Part model, mm, in its own coordinate system. A direction names the side the tool comes from. Coordinates: 2 decimals unless noted, no trailing zeros. Loops run counter-clockwise (first coordinate to the right, second up) from the corner with the lowest first, then second, coordinate; pieces in that order, holes last. Notation, with made-up numbers: M 2,57.5 L 44,57.5 A18 ccw 44,63.5 Z; hole C 53.25,20 d2. An arc over 180 degrees is marked long. Use a Markdown table: item, result. Add a question column.
1) Band-saw the part on A-A (z = 0). List the corners of the cut face in (x, y).
2) Pull direction X, two halves, no side cores. Call faces 1 (the flat face through (-25, -45, 0)), 2 (the flat face through (-12, -70, 0)), 3 (the flat face through (-13, -45, 10)), 4 (the flat face through (0, -32, 0)): released by +X, released by -X, zero draft, split by the parting line, or undercut.
3) Band-saw the part on D-D (z = 5.25). List the corners of the cut face in (x, y), plus the area to 3 significant figures.
4) Band-saw the part on C-C (y = -22.5). List the corners of the cut face in (x, z).
5) Wall check: probe 1 along X at (y, z) = (-73, 0); probe 2 along Z at (x, y) = (-12, -74); probe 3 along Z at (x, y) = (-15.5, -28). Give the ranges that are in metal, low to high. Write a range as from..to.
6) Band-saw the part on B-B (x = -12.5). List the corners of the cut face in (y, z), plus the area to 3 significant figures.
7) Pin check, flat tips, straight feed: pin 1 Ø12 at (x, y) = (-14.5, -48) entering from +Z; pin 2 Ø10 at (y, z) = (-30.5, 0) entering from -X; pin 3 Ø5.5 at (x, z) = (-14, -1) entering from -Y. Stop position of each tip, or through.
8) Tool access for faces 5 (the flat face through (-13, -45, -10)), 6 (the cylindrical face through (-21.286, -75.07, 1.951)), 7 (the flat face through (-10, -80, -9)): list every direction of +Z, -Z, +X, -X, +Y, -Y with a clear straight run to the whole face (end or side of a thin tool).
from build123d import *

# Parameters (mm, degrees)
SKETCH1_R           = 15
BOSS_EXTRUDE1_DEPTH = 50
SKETCH2_W           = 25
SKETCH2_H           = 20
BOSS_EXTRUDE2_DEPTH = 80
SKETCH3_R           = 9
CUT_EXTRUDE2_DEPTH  = 10


with BuildPart() as part:
    # Sketch1 → Boss-Extrude1 (new body)
    with BuildSketch(Plane(origin=(0, 0, 0), x_dir=(0, 0, -1), z_dir=(1, 0, 0))):
        Circle(SKETCH1_R)
    extrude(amount=-BOSS_EXTRUDE1_DEPTH)

    # Sketch2 → Boss-Extrude2 (add)
    with BuildSketch(Plane(origin=(0, 0, 0), x_dir=(1, 0, 0), z_dir=(0, 1, 0))):
        with Locations((-12.5, 0)):
            Rectangle(SKETCH2_W, SKETCH2_H)
    extrude(amount=-BOSS_EXTRUDE2_DEPTH)

    # Sketch3 → Cut-Extrude2 (cut)
    with BuildSketch(Plane.XZ.offset(80)):
        with Locations(Location((-12.5, 0, 0), (0, 0, 270))):
            Circle(SKETCH3_R)
    extrude(amount=-CUT_EXTRUDE2_DEPTH, mode=Mode.SUBTRACT)


solid = part.part
Entries:
| question | item | result |
|---|---|---|
| 1 | outline | M -50,-15 L -25,-15 L -25,-80 L -21.5,-80 L -21.5,-70 L -3.5,-70 L -3.5,-80 L 0,-80 L 0,15 L -50,15 Z |
| 2 | face 1 | released by -X |
| 2 | face 2 | undercut |
| 2 | face 3 | zero draft |
| 2 | face 4 | released by +X |
| 3 | outline | M -50,-14.05 L -25,-14.05 L -25,-80 L -19.81,-80 L -19.81,-70 L -5.19,-70 L -5.19,-80 L 0,-80 L 0,14.05 L -50,14.05 Z |
| 3 | area | 2,910 mm2 |
| 4 | outline | M -25,-10 L 0,-10 L 0,10 L -25,10 Z |
| 5 | probe 1 | -25..-21.5, -3.5..0 |
| 5 | probe 2 | -10..-8.99, 8.99..10 |
| 5 | probe 3 | -10..10 |
| 6 | outline | M -80,-10 L -11.18,-10 A15 ccw long -11.18,10 L -80,10 L -80,9 L -70,9 L -70,-9 L -80,-9 Z |
| 6 | area | 1,850 mm2 |
| 7 | pin 1 | z = 10 |
| 7 | pin 2 | x = -25 |
| 7 | pin 3 | y = -70 |
| 8 | face 5 | -Z, +X, -X, -Y |
| 8 | face 6 | -Y |
| 8 | face 7 | +Z, -Z, +X, -X, -Y |
